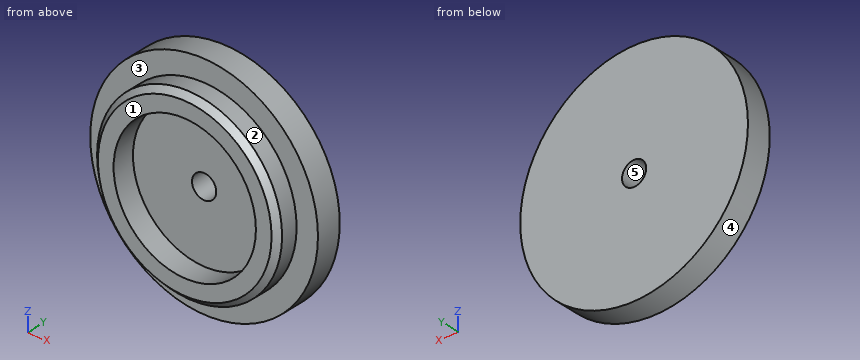
from build123d import *

# Parameters (mm, degrees)
F0_R     = 40
F1_DEPTH = 9
F2_R     = 32.5
F3_DEPTH = 8
F4_R     = 25
F5_DEPTH = 8
F6_R     = 4.25
F7_DEPTH = 25
F8_SIZE  = 2


with BuildPart() as f1:
    # F0 (on Front) → F1 (new body)
    with BuildSketch(Plane.XZ):
        Circle(F0_R)
    extrude(amount=F1_DEPTH)

    # F2 (on face) → F3 (join)
    with BuildSketch(Plane.XZ.offset(9)):
        Circle(F2_R)
    extrude(amount=F3_DEPTH)

    # F4 (on face) → F5 (cut)
    with BuildSketch(Plane.XZ.offset(17)):
        Circle(F4_R)
    extrude(amount=-F5_DEPTH, mode=Mode.SUBTRACT)

    # F6 (on face) → F7 (cut)
    with BuildSketch(Plane.XZ.offset(9)):
        Circle(F6_R)
    extrude(amount=-F7_DEPTH, mode=Mode.SUBTRACT)

    # F8
    f8_edges = [f1.edges().sort_by_distance(p)[0] for p in [
        (-32.5, -17, 0),
    ]]
    chamfer(f8_edges, length=F8_SIZE)


solid = f1.part
Source: CAD feature listing. Evaluate the final solid. Frame: model axes, mm. Face numbers are marked on the shaded views. A direction names the side the tool comes from. Round coordinates to 2 decimals unless told otherwise and drop trailing zeros. Write each loop counter-clockwise with the first axis right and the second up, starting at its lowest first coordinate (ties: lowest second). Pieces come first, ordered by that corner, then holes. Notation, with made-up numbers: M 10,2.5 L 15,2.5 A36 ccw 15,38.5 Z; hole C -22,6.25 d1. An arc over 180 degrees is marked long. One line per item, written item: value. Start each with the question number.
Item 1: Section query D-D (z = 34). Return the cut outline in (x, y).
Item 2: Mould query, pull axis Z, two halves, no side actions, for the marked faces 3, 4 and 5. Classes: pulls with the +Z half, pulls with the -Z half, needs draft (parallel to the pull), parting line crosses it, or undercut.
Item 3: Section query A-A (z = 0). Return the cut outline in (x, y), plus the area to 4 significant figures.
Item 4: Pin query (flat end, axial travel): pin 1 (1 mm diameter, centred on y = -8, z = -23, fed in from +X); pin 2 (5 mm diameter, centred on y = -13.5, z = -21, fed in from -X); pin 3 (3 mm diameter, centred on y = -12.5, z = 27, fed in from +X); pin 4 (7 mm diameter, centred on x = 0, z = 0, fed in from +Y). Return the tip coordinate at first contact, or that it passes through.
Item 5: Section query B-B (x = 0). Return the cut outline in (y, z).
Item 6: Ray query, L1, parallel to Z at x = 0, y = -5; L2, parallel to Z at x = 0, y = -14.5; L3, parallel to Y at x = 19, z = 29.5. Return the intervals inside material, ascending. Write a range as from..to.
Item 7: Set-up query: the marked faces 1 and 2. Return all of +Z, -Z, +X, -X, +Y, -Y with unobstructed straight access to the full face (end or side cutting, diameter ignored); none if empty.
Item 8: Section query C-C (y = -5.5). Return the cut outline in (x, z), plus the area to 3 significant figures.
Result set:
1. outline: M -21.07,-9 L 21.07,-9 L 21.07,0 L -21.07,0 Z
2. face 3: needs draft
2. face 4: parting line crosses it
2. face 5: undercut
3. outline: M -40,-9 L -32.5,-9 L -32.5,-15 L -30.5,-17 L -25,-17 L -25,-9 L -4.25,-9 L -4.25,0 L -40,0 Z; M 4.25,-9 L 25,-9 L 25,-17 L 30.5,-17 L 32.5,-15 L 32.5,-9 L 40,-9 L 40,0 L 4.25,0 Z
3. area: 759.5 mm²
4. pin 1: stops at x = 33.07
4. pin 2: stops at x = -26.72
4. pin 3: stops at x = 20.15
4. pin 4: passes through
5. outline: M -17,-30.5 L -15,-32.5 L -9,-32.5 L -9,-40 L 0,-40 L 0,-4.25 L -9,-4.25 L -9,-25 L -17,-25 Z; M -17,25 L -9,25 L -9,4.25 L 0,4.25 L 0,40 L -9,40 L -9,32.5 L -15,32.5 L -17,30.5 Z
6. L1: z = -40..-4.25, 4.25..40
6. L2: z = -32.5..-25, 25..32.5
6. L3: y = -9..0
7. face 1: +Z, -Z, +X, -X, -Y
7. face 2: -Y
8. outline: C 0,0 d80; hole C 0,0 d8.5
8. area: 4,970 mm²
